from build123d import *

# Parameters (mm, degrees)
F0_W     = 68.209966
F0_H     = 48.351366
F0_R     = 12.668072
F1_DEPTH = 25.4
F2_SIZE2 = 5.08
F2_SIZE  = 5.08
F3_R     = 5.08


with BuildPart() as f1:
    # F0 (on Front) → F1 (new body)
    with BuildSketch(Plane.XZ):
        with Locations((-11.080523, 11.512229)):
            Rectangle(F0_W, F0_H)
        with Locations((-15.992666, 11.620908)):
            Circle(F0_R, mode=Mode.SUBTRACT)
    extrude(amount=F1_DEPTH)

    # F2
    f2_edges = [f1.edges().sort_by_distance(p)[0] for p in [
        (23.02446, -12.7, 35.687912),
        (-45.185506, -12.7, 35.687912),
    ]]
    chamfer(f2_edges, length=F2_SIZE, length2=F2_SIZE2)

    # F3
    f3_edges = [f1.edges().sort_by_distance(p)[0] for p in [
        (-45.185506, -12.7, -12.663454),
        (23.02446, -12.7, -12.663454),
    ]]
    fillet(f3_edges, radius=F3_R)


solid = f1.part
Design review of the part built by this model. Coordinates are the model's own, in mm. Coordinates: 2 decimals unless noted, no trailing zeros. Loops run counter-clockwise (first coordinate to the right, second up) from the corner with the lowest first, then second, coordinate; pieces in that order, holes last. Notation, with made-up numbers: (-23, 35.25) -> (27, 35.25) arc R5 cw to (27, 40.25) -> close; hole circle Ø9 at (43, 71). An arc over 180 degrees is marked (long way). Use a Markdown table: item, result. Add a question column.
Item 1: We need section A-A, the plane z = 1.5. Write out the cut boundary in (x, y).
Item 2: The part is to be moulded in two halves that separate along Z. For faces 1 (the flat face through (-42.61, -12.522, 33.183)), 2 (the flat face through (23.024, -13, 11)), 3 (the flat face through (-11, -13, -12.663)), 4 (the cylindrical face through (-26.046, -12.522, 3.913)), say which applies: +Z half, -Z half, draft (parallel to the pull), parting line (faces both ways), or undercut.
Item 3: We need section D-D, the plane z = 32.5. Write out the cut boundary in (x, y), and give its area (3 significant figures).
Item 4: We need section C-C, the plane y = -9.5. Write out the cut boundary in (x, z).
Item 5: We need section B-B, the plane x = -12.5. Write out the cut boundary in (y, z), and give its area (3 significant figures).
Item 6: Wall thickness on L1, parallel to X at y = -16.75, z = 0.5; L2, parallel to X at y = -13, z = 6; L3, parallel to X at y = -15, z = 31: over which ranges is each line inside the solid? List them lowest first. Write a range as from..to.
Item 7: Clearance check with a flat-ended pin moving along its axis: P1, Ø20.5, axis at x = -15.99, z = 11.62, coming from the +Y side. State where the tip first meets the part, or that it passes through.
Numbers:
| question | item | result |
|---|---|---|
| 1 | outline | (-45.19, -25.4) -> (-23.61, -25.4) -> (-23.61, 0) -> (-45.19, 0) -> close; (-8.37, -25.4) -> (23.02, -25.4) -> (23.02, 0) -> (-8.37, 0) -> close |
| 2 | face 1 | +Z half |
| 2 | face 2 | draft |
| 2 | face 3 | -Z half |
| 2 | face 4 | undercut |
| 3 | outline | (-43.29, -25.4) -> (21.13, -25.4) -> (21.13, 0) -> (-43.29, 0) -> close |
| 3 | area | 1,640 mm^2 |
| 4 | outline | (-45.19, -7.58) arc R5.08 ccw to (-40.11, -12.66) -> (17.94, -12.66) arc R5.08 ccw to (23.02, -7.58) -> (23.02, 30.61) -> (17.94, 35.69) -> (-40.11, 35.69) -> (-45.19, 30.61) -> close; hole circle Ø25.34 at (-15.99, 11.62) |
| 5 | outline | (-25.4, -12.66) -> (0, -12.66) -> (0, -0.56) -> (-25.4, -0.56) -> close; (-25.4, 23.8) -> (0, 23.8) -> (0, 35.69) -> (-25.4, 35.69) -> close |
| 5 | area | 610 mm^2 |
| 6 | L1 | x = -45.19..-22.06, -9.93..23.02 |
| 6 | L2 | x = -45.19..-27.35, -4.64..23.02 |
| 6 | L3 | x = -44.79..22.63 |
| 7 | P1 | passes through |
